Print and shaded views of the part. All mm, measured from the part's lowest x, y and z. A direction names the side the tool comes from. Round coordinates to 2 decimals unless told otherwise and drop trailing zeros. Order: outer loops, then holes, each group sorted by start corner. A loop starts at its lowest first (then second) coordinate and runs counter-clockwise, first axis right, second up.
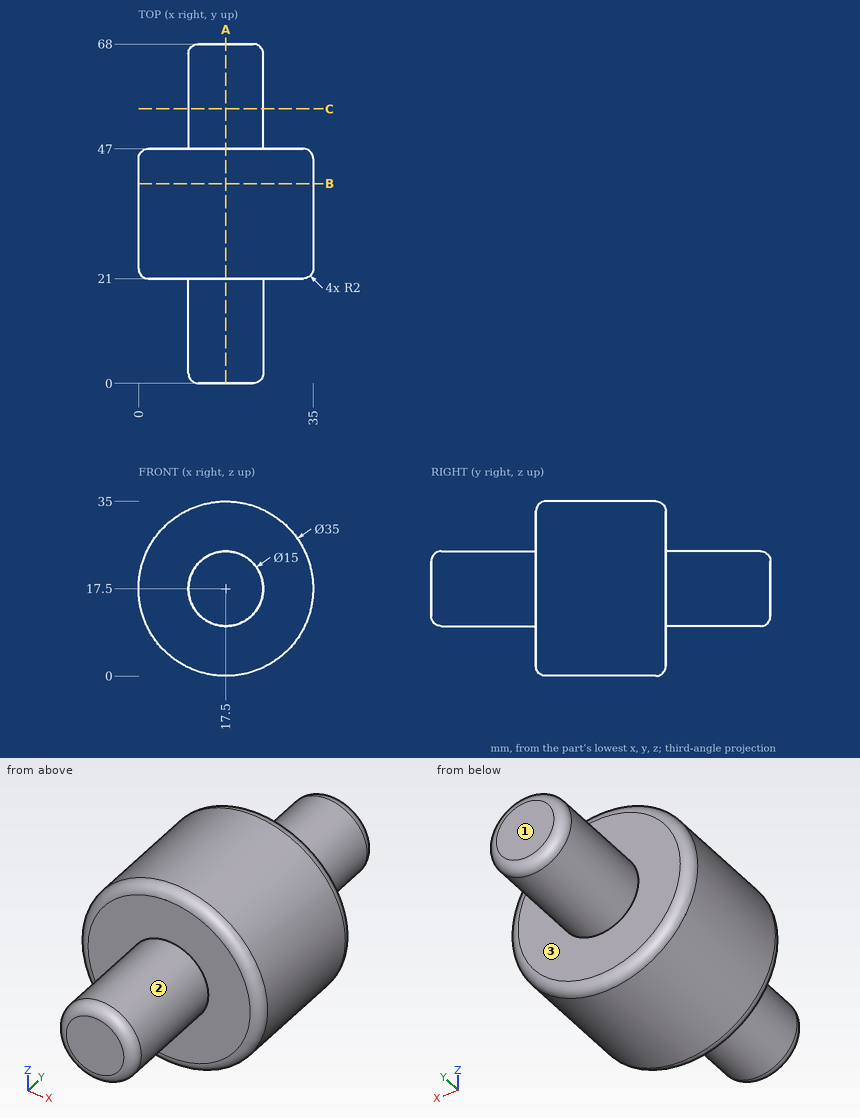
1. Pin check, flat tips, straight feed: P1, Ø4, axis at x = 19, y = 17.5, coming from the -Z side; P2, Ø4, axis at y = 26, z = 5.5, coming from the -X side; P3, Ø3, axis at x = 13.5, z = 10, coming from the +Y side. Stop position of each tip, or through.
2. Cut at C-C, the plane y = 55. Write the cut outline in (x, z), and give its area (3 significant figures).
3. Tool access for the marked faces 1, 2 and 3: list every direction of +Z, -Z, +X, -X, +Y, -Y with a clear straight run to the whole face (end or side of a thin tool).
4. Drill centre lines: line 1 (Y direction, x = 21.5, z = 25); line 2 (X direction, y = 24.5, z = 25); line 3 (X direction, y = 31, z = 14). Where is each one in solid material? Low to high.
5. Cut at B-B, the plane y = 40. Write the cut outline in (x, z), and give its area (3 significant figures).
6. Cut at A-A, the plane x = 17.5. Write the cut outline in (y, z).
Outcome:
1. P1: stops at z = 10
1. P2: stops at x = 3.14
1. P3: stops at y = 67.32
2. outline: circle Ø15 at (17.5, 17.5)
2. area: 177 mm2
3. face 1: +Z, -Z, +X, -X, +Y
3. face 2: -Y
3. face 3: +Y
4. line 1: y = 21 to 47
4. line 2: x = 1.69 to 33.31
4. line 3: x = 0.35 to 34.65
5. outline: circle Ø35 at (17.5, 17.5)
5. area: 962 mm2
6. outline: (0, 12) arc R2 ccw to (2, 10) - (21, 10) - (21, 2) arc R2 ccw to (23, 0) - (45, 0) arc R2 ccw to (47, 2) - (47, 10) - (66, 10) arc R2 ccw to (68, 12) - (68, 23) arc R2 ccw to (66, 25) - (47, 25) - (47, 33) arc R2 ccw to (45, 35) - (23, 35) arc R2 ccw to (21, 33) - (21, 25) - (2, 25) arc R2 ccw to (0, 23) - close
